from build123d import *

# Parameters (mm, degrees)
F2_R     = 4.1
F3_DEPTH = 50
F4_R     = 3
F5_DEPTH = 50
F7_R     = 1
F8_R     = 50
F9_DEPTH = 50


# Not quite as in the source:
# - a fillet or chamfer that OpenCascade refuses, or shapes differently, is made with other operations: its cross-section is extruded or revolved along the edge and cut away or added
# - a feature names something its author has since deleted; it is built from what else it names


with BuildPart() as f1:
    # F0 (on Top) → F1 (revolve)
    with BuildSketch(Plane.XY):
        Polygon((-7, 49), (-7, 32.05), (0, 32.05), (0, 51), (6.6556592449, 51), (12.5, 62.9584203143), (12.5, 80), (5.5, 80), (5.5, 62.3), (-0.5, 62.3), align=None)
    revolve(axis=Axis((-3.5, 0, 0), (1, 0, 0)))

    # F2 (on Right) → F3 (cut, symmetric)
    with BuildSketch(Plane.YZ):
        with Locations((-40, 0)):
            Circle(F2_R)
        with Locations((-20, -34.6410161514)):
            Circle(F2_R)
        with Locations((20, -34.6410161514)):
            Circle(F2_R)
        with Locations((40, 0)):
            Circle(F2_R)
        with Locations((20, 34.6410161514)):
            Circle(F2_R)
        with Locations((-20, 34.6410161514)):
            Circle(F2_R)
    extrude(amount=F3_DEPTH, both=True, mode=Mode.SUBTRACT)

    # F4 (on face) → F5 (cut, symmetric)
    with BuildSketch(Plane(origin=(5.5, 0, 0), x_dir=(0, -1, 0), z_dir=(-1, 0, 0))):
        with Locations((35.75, 61.9208163706)):
            Circle(F4_R)
        with Locations((-35.75, 61.9208163706)):
            Circle(F4_R)
        with Locations((-71.5, 0)):
            Circle(F4_R)
        with Locations((-35.75, -61.9208163706)):
            Circle(F4_R)
        with Locations((35.75, -61.9208163706)):
            Circle(F4_R)
        with Locations((71.5, 0)):
            Circle(F4_R)
    extrude(amount=F5_DEPTH, both=True, mode=Mode.SUBTRACT)

    # F6: chamfer of 4 on 6 edges, made by hand

    # F6_s1 → F6_t2 (revolve, cut)
    with BuildSketch(Plane.XY.offset(34.6410161514)):
        Polygon((-7, 28.1), (-3, 24.1), (-7, 24.1), align=None)
    revolve(axis=Axis((-7, 20, 34.6410161514), (1, 0, 0)), mode=Mode.SUBTRACT)

    # F6_s3 → F6_t4 (revolve, cut)
    with BuildSketch(Plane.XY.offset(34.6410161514)):
        Polygon((-7, -11.9), (-3, -15.9), (-7, -15.9), align=None)
    revolve(axis=Axis((-7, -20, 34.6410161514), (1, 0, 0)), mode=Mode.SUBTRACT)

    # F6_s5 → F6_t6 (revolve, cut)
    with BuildSketch(Plane.XY):
        Polygon((-7, -31.9), (-3, -35.9), (-7, -35.9), align=None)
    revolve(axis=Axis((-7, -40, 0), (1, 0, 0)), mode=Mode.SUBTRACT)

    # F6_s7 → F6_t8 (revolve, cut)
    with BuildSketch(Plane.XY.offset(-34.6410161514)):
        Polygon((-7, -11.9), (-3, -15.9), (-7, -15.9), align=None)
    revolve(axis=Axis((-7, -20, -34.6410161514), (1, 0, 0)), mode=Mode.SUBTRACT)

    # F6_s9 → F6_t10 (revolve, cut)
    with BuildSketch(Plane.XY.offset(-34.6410161514)):
        Polygon((-7, 28.1), (-3, 24.1), (-7, 24.1), align=None)
    revolve(axis=Axis((-7, 20, -34.6410161514), (1, 0, 0)), mode=Mode.SUBTRACT)

    # F6_s11 → F6_t12 (revolve, cut)
    with BuildSketch(Plane.XY):
        Polygon((-7, 48.1), (-3, 44.1), (-7, 44.1), align=None)
    revolve(axis=Axis((-7, 40, 0), (1, 0, 0)), mode=Mode.SUBTRACT)

    # F7
    f7_edges = [f1.edges().sort_by_distance(p)[0] for p in [
        (0, -51, 0),
    ]]
    fillet(f7_edges, radius=F7_R)

    # F8 (on face) → F9 (cut, symmetric)
    with BuildSketch(Plane(origin=(5.5, 0, 0), x_dir=(0, -1, 0), z_dir=(-1, 0, 0))):
        with Locations((0, 113)):
            Circle(F8_R)
        with Locations((-97.8608706276, 56.5)):
            Circle(F8_R)
        with Locations((-97.8608706276, -56.5)):
            Circle(F8_R)
        with Locations((0, -113)):
            Circle(F8_R)
        with Locations((97.8608706276, -56.5)):
            Circle(F8_R)
        with Locations((97.8608706276, 56.5)):
            Circle(F8_R)
    extrude(amount=F9_DEPTH, both=True, mode=Mode.SUBTRACT)


solid = f1.part
Geometry: final body of the model. Coordinates: model frame, mm. Give positions to 0.01 mm unless a question says otherwise; leave off trailing zeros. Order: outer loops, then holes, each group sorted by start corner. A loop starts at its lowest first (then second) coordinate and runs counter-clockwise, first axis right, second up. Notation, with made-up numbers: (46.5, 30.5) - (60.5, 30.5) arc R25 ccw to (60.5, 46.5) - close; hole circle Ø9 at (44, -30.75). An arc over 180 degrees is marked (long way). Use CSV: the item, a comma, the result in double quotes.
1. Mould query, pull axis Y, two halves, no side actions, for faces 1 (the face through (12.5, 18.151, 60.442)), 2 (the face through (8.951, 54.795, 31.096)), 3 (the face through (9, 73.9, -1.8)), 4 (the face through (8.951, -54.328, 31.906)). Classes: +Y half, -Y half, draft (parallel to the pull), parting line (faces both ways), or undercut.
Answers below:
face 1,"draft"
face 2,"+Y half"
face 3,"undercut"
face 4,"-Y half"
2. Section query A-A (y = 0). Output: boundary loops of the cut face in (x, z), plus the area to 3 significant figures.
Answers below:
outline,"(-7, -49) - (-0.5, -62.3) - (5.5, -62.3) - (5.5, -63) - (12.5, -63) - (12.5, -62.96) - (6.66, -51) - (1, -51) arc R1 cw to (0, -50) - (0, -32.05) - (-7, -32.05) - close; (-7, 32.05) - (0, 32.05) - (0, 50) arc R1 cw to (1, 51) - (6.66, 51) - (12.5, 62.96) - (12.5, 63) - (5.5, 63) - (5.5, 62.3) - (-0.5, 62.3) - (-7, 49) - close"
area,"560 mm2"
3. Section query C-C (y = -71.5). Output: boundary loops of the cut face in (x, z).
Answers below:
outline,"(5.5, -14.01) - (12.5, -14.01) - (12.5, -3) - (5.5, -3) - close; (5.5, 3) - (12.5, 3) - (12.5, 14.01) - (5.5, 14.01) - close"
4. Section query D-D (x = 10). Output: boundary loops of the cut face in (y, z).
Answers below:
outline,"(-79.37, -10.05) arc R50 cw to (-48.38, -63.71) arc R80 ccw to (-30.98, -73.76) arc R50 cw to (30.98, -73.76) arc R80 ccw to (48.38, -63.71) arc R50 cw to (79.37, -10.05) arc R80 ccw to (79.37, 10.05) arc R50 cw to (48.38, 63.71) arc R80 ccw to (30.98, 73.76) arc R50 cw to (-30.98, 73.76) arc R80 ccw to (-48.38, 63.71) arc R50 cw to (-79.37, 10.05) arc R80 ccw to start; hole circle Ø6 at (-71.5, 0); hole circle Ø115.69 at (0, 0); hole circle Ø6 at (-35.75, -61.92); hole circle Ø6 at (-35.75, 61.92); hole circle Ø6 at (35.75, -61.92); hole circle Ø6 at (35.75, 61.92); hole circle Ø6 at (71.5, 0)"
5. Material intervals for line 1 along Z through (x, y) = (-1.25, 20); line 2 along X through (y, z) = (30.5, -14.5); line 3 along Z through (x, y) = (11.25, 25), sorted ascending. Write a range as from..to.
Answers below:
line 1,"-57.38..-38.74, -30.54..-25.04, 25.04..30.54, 38.74..57.38"
line 2,"-7..0"
line 3,"-69.7..-54.98, 54.98..69.7"
6. Section query B-B (x = -5). Output: boundary loops of the cut face in (y, z).
Answers below:
outline,"circle Ø106.18 at (0, 0); hole circle Ø12.2 at (-40, 0); hole circle Ø64.1 at (0, 0); hole circle Ø12.2 at (-20, -34.64); hole circle Ø12.2 at (-20, 34.64); hole circle Ø12.2 at (20, -34.64); hole circle Ø12.2 at (20, 34.64); hole circle Ø12.2 at (40, 0)"
7. Contact query for flat-ended pins moving along their axis: pin 1 (10 mm diameter, centred on x = 3.5, z = -55.5, fed in from +Y); pin 2 (13 mm diameter, centred on y = -40, z = 0, fed in from +X); pin 3 (1.5 mm diameter, centred on x = 4.5, y = -21.5, fed in from +Z). Output: stop coordinate, or through.
Answers below:
pin 1,"y = 48.17"
pin 2,"x = 0"
pin 3,"z = 58.74"
